Read the model definition and answer for the solid it produces. Units are mm, in the model's axes. A direction names the side the tool comes from. Coordinates: 2 decimals unless noted, no trailing zeros. Write each loop counter-clockwise with the first axis right and the second up, starting at its lowest first coordinate (ties: lowest second). Pieces come first, ordered by that corner, then holes.
Item 1: Straight lines are drawn through the part: probe 1 along Y at (x, z) = (0, 2.4); probe 2 along X at (y, z) = (-0.5, 2.7); probe 3 along X at (y, z) = (-1, 0.55). For each, find the intervals that lie inside material, in ascending order.
Item 2: Section A-A (x = 6) is taken. Give the vertices of the cut face in (y, z), then the cut area to 3 significant figures.
Item 3: Each of these flat-tipped pins is pushed along its axis until it touches: P1, Ø10, axis at x = 1.5, y = -1.5, coming from the +Z side; P2, Ø1, axis at y = 5, z = 0.5, coming from the -X side; P3, Ø1.5, axis at y = 1, z = 2.5, coming from the -X side. Where does it stop, or does it pass through?
Item 4: Determine the mould class of faces 3 (the face through (9, -2, 0)), 4 (the face through (9.3, 0, 0.75)) for opening direction Y: released by +Y, released by -Y, zero draft, split by the parting line, or undercut.
Item 5: Section C-C (y = 6.5) is taken. Give the vertices of the cut face in (x, z), then the cut area to 3 significant figures.
Item 6: A tool of negligible diameter and unlimited length cuts with its end or side. For faces 1 (the face through (9, -2, 3)), 2 (the face through (9.3, 0, 2.25)), from which of +Z, -Z, +X, -X, +Y, -Y can it reach the whole face along a straight path? Write none if from no direction.
Item 7: Section B-B (y = 1.5) is taken. Give the vertices of the cut face in (x, z).
Item 8: Section D-D (z = 1) is taken. Give the vertices of the cut face in (x, y).
from build123d import *

# Parameters (mm, degrees)
F0_R         = 10
F0_R_2       = 9.05
F1_DEPTH     = 3
F3_DEPTH     = 25
F4_T4_DEPTH  = 5.0690329252
F4_S5_R      = 10
F4_T6_DEPTH  = 4
F4_S7_R      = 9.05
F4_T8_DEPTH  = 4
F4_T12_DEPTH = 5.0690329252
F4_S13_R     = 10
F4_T14_DEPTH = 4
F4_S15_R     = 9.05
F4_T16_DEPTH = 4
F4_T20_DEPTH = 5.0814545551
F4_S21_R     = 10
F4_T22_DEPTH = 4
F4_S23_R     = 9.05
F4_T24_DEPTH = 4
F4_T28_DEPTH = 5.0814545551
F4_S29_R     = 10
F4_T30_DEPTH = 4
F4_S31_R     = 9.05
F4_T32_DEPTH = 4


# Not quite as in the source:
# - a fillet or chamfer that OpenCascade refuses, or shapes differently, is made with other operations: its cross-section is extruded or revolved along the edge and cut away or added


with BuildPart() as f1:
    # F0 (on Top) → F1 (new body)
    with BuildSketch(Plane.XY):
        Circle(F0_R)
        with Locations((-0.0741272524, -0.0176765498)):
            Circle(F0_R_2, mode=Mode.SUBTRACT)
    extrude(amount=F1_DEPTH)

    # F2 (on Right) → F3 (cut)
    with BuildSketch(Plane.YZ):
        Polygon((3, 0.75), (3, 2.25), (-3, 2.25), (-3, 0.75), (0, 0.75), align=None)
    extrude(amount=F3_DEPTH, mode=Mode.SUBTRACT)

    # F4: fillet of radius 0.8 on 4 edges, made by hand


with BuildPart() as f4_tool2:
    # F4_s3 → F4_t4 (new body)
    with BuildSketch(Plane.YZ.offset(6.4703590889)):
        with BuildLine():
            ThreePointArc((-3, 1.45), (-2.7656854249, 2.0156854249), (-2.2, 2.25))
            Line((-2.2, 2.25), (-3, 2.25))
            Line((-3, 2.25), (-3, 1.45))
        make_face()
    extrude(amount=F4_T4_DEPTH)

    # F4_s5 → F4_t6 (intersect, symmetric)
    with BuildSketch(Plane.XY.offset(1.9)):
        Circle(F4_S5_R)
    extrude(amount=F4_T6_DEPTH, both=True, mode=Mode.INTERSECT)

    # F4_s7 → F4_t8 (cut, symmetric)
    with BuildSketch(Plane.XY.offset(1.9)):
        with Locations((-0.0741272524, -0.0176765498)):
            Circle(F4_S7_R)
    extrude(amount=F4_T8_DEPTH, both=True, mode=Mode.SUBTRACT)


with BuildPart() as f1_1:
    add(f1.part)

    # F4_t1: union F4_tool2
    add(f4_tool2.part)


with BuildPart() as f4_tool10:
    # F4_s11 → F4_t12 (new body)
    with BuildSketch(Plane.YZ.offset(6.4703590889)):
        with BuildLine():
            ThreePointArc((-2.2, 0.75), (-2.7656854249, 0.9843145751), (-3, 1.55))
            Line((-3, 1.55), (-3, 0.75))
            Line((-3, 0.75), (-2.2, 0.75))
        make_face()
    extrude(amount=F4_T12_DEPTH)

    # F4_s13 → F4_t14 (intersect, symmetric)
    with BuildSketch(Plane.XY.offset(1.1)):
        Circle(F4_S13_R)
    extrude(amount=F4_T14_DEPTH, both=True, mode=Mode.INTERSECT)

    # F4_s15 → F4_t16 (cut, symmetric)
    with BuildSketch(Plane.XY.offset(1.1)):
        with Locations((-0.0741272524, -0.0176765498)):
            Circle(F4_S15_R)
    extrude(amount=F4_T16_DEPTH, both=True, mode=Mode.SUBTRACT)


with BuildPart() as f1_2:
    add(f1_1.part)

    # F4_t9: union F4_tool10
    add(f4_tool10.part)


with BuildPart() as f4_tool18:
    # F4_s19 → F4_t20 (new body)
    with BuildSketch(Plane.YZ.offset(6.457937459)):
        with BuildLine():
            ThreePointArc((2.2, 2.25), (2.7656854249, 2.0156854249), (3, 1.45))
            Line((3, 1.45), (3, 2.25))
            Line((3, 2.25), (2.2, 2.25))
        make_face()
    extrude(amount=F4_T20_DEPTH)

    # F4_s21 → F4_t22 (intersect, symmetric)
    with BuildSketch(Plane.XY.offset(1.9)):
        Circle(F4_S21_R)
    extrude(amount=F4_T22_DEPTH, both=True, mode=Mode.INTERSECT)

    # F4_s23 → F4_t24 (cut, symmetric)
    with BuildSketch(Plane.XY.offset(1.9)):
        with Locations((-0.0741272524, -0.0176765498)):
            Circle(F4_S23_R)
    extrude(amount=F4_T24_DEPTH, both=True, mode=Mode.SUBTRACT)


with BuildPart() as f1_3:
    add(f1_2.part)

    # F4_t17: union F4_tool18
    add(f4_tool18.part)


with BuildPart() as f4_tool26:
    # F4_s27 → F4_t28 (new body)
    with BuildSketch(Plane.YZ.offset(6.457937459)):
        with BuildLine():
            ThreePointArc((2.2, 0.75), (2.7656854249, 0.9843145751), (3, 1.55))
            Line((3, 1.55), (3, 0.75))
            Line((3, 0.75), (2.2, 0.75))
        make_face()
    extrude(amount=F4_T28_DEPTH)

    # F4_s29 → F4_t30 (intersect, symmetric)
    with BuildSketch(Plane.XY.offset(1.1)):
        Circle(F4_S29_R)
    extrude(amount=F4_T30_DEPTH, both=True, mode=Mode.INTERSECT)

    # F4_s31 → F4_t32 (cut, symmetric)
    with BuildSketch(Plane.XY.offset(1.1)):
        with Locations((-0.0741272524, -0.0176765498)):
            Circle(F4_S31_R)
    extrude(amount=F4_T32_DEPTH, both=True, mode=Mode.SUBTRACT)


with BuildPart() as f1_4:
    add(f1_3.part)

    # F4_t25: union F4_tool26
    add(f4_tool26.part)


solid = f1_4.part
Established:
1. probe 1: y = -10 to -9.07, 9.03 to 10
1. probe 2: x = -9.99 to -9.11, 8.96 to 9.99
1. probe 3: x = -9.95 to -9.07, 8.92 to 9.95
2. outline: (-8, 0) - (-6.73, 0) - (-6.73, 3) - (-8, 3) - close; (6.69, 0) - (8, 0) - (8, 3) - (6.69, 3) - close
2. area: 7.75 mm2
3. P1: passes through
3. P2: stops at x = -8.93
3. P3: stops at x = -10
4. face 3: zero draft
4. face 4: undercut
5. outline: (-7.6, 0) - (-6.35, 0) - (-6.35, 3) - (-7.6, 3) - close; (6.2, 0) - (7.6, 0) - (7.6, 3) - (6.2, 3) - close
5. area: 7.92 mm2
6. face 1: +Z, +X, -X, +Y, -Y
6. face 2: +X
7. outline: (-9.89, 0) - (-9, 0) - (-9, 3) - (-9.89, 3) - close; (8.85, 0) - (9.89, 0) - (9.89, 0.75) - (8.85, 0.75) - close; (8.85, 2.25) - (9.89, 2.25) - (9.89, 3) - (8.85, 3) - close
8. outline: (8.53, 2.78) - (9.61, 2.78) arc R10 ccw (long way) to (9.61, -2.78) - (8.54, -2.78) arc R9.05 cw (long way) to start
